Read the model definition and answer for the solid it produces. Units are mm, in the model's axes. A direction names the side the tool comes from. Coordinates: 2 decimals unless noted, no trailing zeros. Write each loop counter-clockwise with the first axis right and the second up, starting at its lowest first coordinate (ties: lowest second). Pieces come first, ordered by that corner, then holes.
1) The part is cut by section D-D (z = -23). Determine the outline of the cut face in (x, y), then the cut area to 3 significant figures.
2) The part is cut by section C-C (y = 53.5). Determine the outline of the cut face in (x, z), then the cut area to 3 significant figures.
3) Which of the six approach directions +Z, -Z, +X, -X, +Y, -Y give full straight-line access (tool end or side, diameter ignored) to faces 1 (the face through (-19.05, 72, -37)), 2 (the face through (37, 72, -19.05)), 3 (the face through (-19.05, 72, 37)), 4 (the face through (-26.5, 139.7, -26.9)), 5 (the face through (-41, 135, 3.81))?
4) The part is cut by section A-A (z = 0). Determine the outline of the cut face in (x, y).
5) The part is cut by section B-B (x = 0). Determine the outline of the cut face in (y, z).
6) Find the intervals of material crossed by line 1 (Y direction, x = -36.5, z = -10); line 2 (Y direction, x = 22.5, z = -9); line 3 (Z direction, x = -26.5, y = 96), in increasing order.
7) Determine the mould class of faces 6 (the face through (19.05, 72, -37)), 7 (the face through (3.81, 135, 41)) for opening direction Z: +Z half, -Z half, draft (parallel to the pull), parting line (faces both ways), or undercut.
8) Each of these flat-tipped pins is pushed along its axis until it touches: pin 1 Ø9.5 at (y, z) = (90.5, -36.5) entering from -X; pin 2 Ø1.1 at (y, z) = (133.5, -42) entering from +X; pin 3 Ø4 at (y, z) = (133.5, -42) entering from -X. Where does it stop, or does it pass through?
from build123d import *

# Parameters (mm, degrees)
SKETCH1_R           = 45
BOSS_EXTRUDE3_DEPTH = 139.7
SHELL2_T            = -7.62
SKETCH15_W          = 38.1
SKETCH15_H          = 116.84
CUT_EXTRUDE3_DEPTH  = 12.7
CIRPATTERN4_COUNT   = 4
SKETCH14_W          = 3.81
SKETCH14_H          = 6.985
CUT_EXTRUDE2_DEPTH  = 12.7
CIRPATTERN3_COUNT   = 4


with BuildPart() as part:
    # Sketch1 → Boss-Extrude3 (new body)
    with BuildSketch(Plane(origin=(0, 0, 0), x_dir=(1, 0, 0), z_dir=(0, 1, 0))):
        with Locations(Location((0, 0, 0), (0, 0, 270))):
            Circle(SKETCH1_R)
    extrude(amount=BOSS_EXTRUDE3_DEPTH)

    # Shell2
    shell2_openings = [part.faces().sort_by_distance(p)[0] for p in [
        (0, 139.7, 0),
    ]]
    offset(amount=SHELL2_T, openings=shell2_openings, kind=Kind.INTERSECTION)

    # Sketch15 → Cut-Extrude3 (cut)
    with BuildSketch(Plane(origin=(45, 0, 0), x_dir=(0, 0, -1), z_dir=(1, 0, 0))):
        with Locations((0, 72.39)):
            Rectangle(SKETCH15_W, SKETCH15_H)
    cut_extrude3 = extrude(amount=-CUT_EXTRUDE3_DEPTH, mode=Mode.SUBTRACT)

    # CirPattern4: Cut-Extrude3 ×4 about axis
    cirpattern4_axis = Axis((0, 0, 0), (0, 1, 0))
    for i in range(1, CIRPATTERN4_COUNT):
        add(cut_extrude3.rotate(cirpattern4_axis, i * 360 / CIRPATTERN4_COUNT), mode=Mode.SUBTRACT)

    # Sketch14 → Cut-Extrude2 (cut)
    with BuildSketch(Plane(origin=(0, 142.24, 0), x_dir=(1, 0, 0), z_dir=(0, 1, 0))):
        with Locations((-41.106583324, -0.3175)):
            Rectangle(SKETCH14_W, SKETCH14_H)
    cut_extrude2 = extrude(amount=-CUT_EXTRUDE2_DEPTH, mode=Mode.SUBTRACT)

    # CirPattern3: Cut-Extrude2 ×4 about axis
    cirpattern3_axis = Axis((0, 0, 0), (0, 1, 0))
    for i in range(1, CIRPATTERN3_COUNT):
        add(cut_extrude2.rotate(cirpattern3_axis, i * 360 / CIRPATTERN3_COUNT), mode=Mode.SUBTRACT)


solid = part.part
Reported:
1. outline: (-38.68, 0) - (38.68, 0) - (38.68, 139.7) - (29.47, 139.7) - (29.47, 7.62) - (-29.47, 7.62) - (-29.47, 139.7) - (-38.68, 139.7) - close
1. area: 3,020 mm2
2. outline: (-40.77, -19.05) arc R45 ccw to (-19.05, -40.77) - (-19.05, -32.3) - (-18.81, -32.3) arc R37.38 cw to (-32.3, -18.81) - (-32.3, -19.05) - close; (-40.77, 19.05) - (-32.3, 19.05) - (-32.3, 18.81) arc R37.38 cw to (-18.81, 32.3) - (-19.05, 32.3) - (-19.05, 40.77) arc R45 ccw to start; (18.81, -32.3) - (19.05, -32.3) - (19.05, -40.77) arc R45 ccw to (40.77, -19.05) - (32.3, -19.05) - (32.3, -18.81) arc R37.38 cw to start; (18.81, 32.3) arc R37.38 cw to (32.3, 18.81) - (32.3, 19.05) - (40.77, 19.05) arc R45 ccw to (19.05, 40.77) - (19.05, 32.3) - close
2. area: 764 mm2
3. face 1: -Z
3. face 2: +X
3. face 3: +Z
3. face 4: +Z, -Z, +X, -X, +Y
3. face 5: +Y
4. outline: (-45, 0) - (45, 0) - (45, 13.97) - (37.38, 13.97) - (37.38, 7.62) - (-37.38, 7.62) - (-37.38, 13.97) - (-45, 13.97) - close; (-45, 130.81) - (-43.01, 130.81) - (-43.01, 139.7) - (-45, 139.7) - close; (-39.2, 130.81) - (-37.38, 130.81) - (-37.38, 139.7) - (-39.2, 139.7) - close; (37.38, 130.81) - (39.2, 130.81) - (39.2, 139.7) - (37.38, 139.7) - close; (43.01, 130.81) - (45, 130.81) - (45, 139.7) - (43.01, 139.7) - close
5. outline: (0, -45) - (13.97, -45) - (13.97, -37.38) - (7.62, -37.38) - (7.62, 37.38) - (13.97, 37.38) - (13.97, 45) - (0, 45) - close; (130.81, -45) - (139.7, -45) - (139.7, -43.01) - (130.81, -43.01) - close; (130.81, -39.2) - (139.7, -39.2) - (139.7, -37.38) - (130.81, -37.38) - close; (130.81, 37.38) - (139.7, 37.38) - (139.7, 39.2) - (130.81, 39.2) - close; (130.81, 43.01) - (139.7, 43.01) - (139.7, 45) - (130.81, 45) - close
6. line 1: y = 0 to 13.97, 130.81 to 139.7
6. line 2: y = 0 to 7.62
6. line 3: z = -36.37 to -26.36, 26.36 to 36.37
7. face 6: draft
7. face 7: undercut
8. pin 1: stops at x = -31.89
8. pin 2: stops at x = 17.52
8. pin 3: stops at x = -20.62
